```python
from build123d import *

# Parameters (mm, degrees)
EXTRUDE_1_DEPTH = 90
SKETCH_4_R      = 1.5
EXTRUDE_2_DEPTH = 6
M3X0_5_1_D      = 2.5
M3X0_5_1_DEPTH  = 7.5
M3X0_5_1_TIP    = 0.751075774


with BuildPart() as part:
    # 草圖1 → 填料-伸長1 (new body)
    with BuildSketch(Plane.XY):
        Polygon((-1.443375673, 2.5), (-2.886751346, 0), (-1.443375673, -2.5), (1.443375673, -2.5), (2.886751346, 0), (1.443375673, 2.5), align=None)
    extrude(amount=EXTRUDE_1_DEPTH)

    # 草圖4 → 填料-伸長2 (add)
    with BuildSketch(Plane(origin=(0, 0, 0), x_dir=(-1, 0, 0), z_dir=(0, 0, -1))):
        Circle(SKETCH_4_R)
    extrude(amount=EXTRUDE_2_DEPTH)

    # M3x0.5 螺紋孔1
    with Locations(Plane.XY.offset(90)):
        with Locations((0, 0)):
            Hole(M3X0_5_1_D / 2, depth=M3X0_5_1_DEPTH)
            with Locations((0, 0, -(M3X0_5_1_DEPTH + M3X0_5_1_TIP / 2))):  # 118° drill point
                Cone(0, M3X0_5_1_D / 2, M3X0_5_1_TIP, mode=Mode.SUBTRACT)


solid = part.part
```
Verification items for the finished model (mm, model axes). A direction names the side the tool comes from. Give positions to 0.01 mm unless a question says otherwise; leave off trailing zeros. Loops run counter-clockwise (first coordinate to the right, second up) from the corner with the lowest first, then second, coordinate; pieces in that order, holes last.
1. Section check A-A, the plane z = 78.5. Enter the section's corners in (x, y), then the cut area to 3 significant figures.
2. Set-up check for faces 1 (the flat face through (1.24, 1.15, 0)), 2 (the flat face through (0, 2.5, 44)): record each of +Z, -Z, +X, -X, +Y, -Y from which the full face is reachable in a straight line by a thin tool's end or side.
3. Thickness scan on line 1 (X direction, y = 0, z = 88.75); line 2 (Y direction, x = 0, z = 85); line 3 (Z direction, x = -1.55, y = -1.1). Record the ranges inside material, lowest first.
4. Mould release check, pull along Y, two halves, no side actions. Record for faces 3 (the flat face through (-2.175, -1.233, 44.37)), 4 (the flat face through (0, 0, -6)), 5 (the cylindrical face through (0.27, -1.22, 86.2)), 6 (the conical face through (-0.05, -0.21, 81.88)): released by +Y, released by -Y, zero draft, split by the parting line, or undercut.
5. Go/stop test with flat-tipped pins: pin 1 Ø1.5 at (x, y) = (1, 0) entering from +Z; pin 2 Ø2 at (y, z) = (-1.5, 26) entering from -X. Record where each tip stops, or that it passes through.
Geometry says:
1. outline: (-2.89, 0) - (-1.44, -2.5) - (1.44, -2.5) - (2.89, 0) - (1.44, 2.5) - (-1.44, 2.5) - close
1. area: 21.7 mm2
2. face 1: -Z
2. face 2: +Z, -Z, +X, -X, +Y
3. line 1: x = -2.89 to -1.25, 1.25 to 2.89
3. line 2: y = -2.5 to -1.25, 1.25 to 2.5
3. line 3: z = 0 to 90
4. face 3: released by -Y
4. face 4: zero draft
4. face 5: undercut
4. face 6: undercut
5. pin 1: stops at z = 90
5. pin 2: stops at x = -2.6
